from build123d import *

# Parameters (mm, degrees)
EXTRUDE_1_DEPTH = 2
FILLET_1_R      = 2


with BuildPart() as part:
    # 草图1 → 凸台-拉伸1 (new body)
    with BuildSketch(Plane.XY):
        Polygon((-8.301811847, -11.701358885), (-3.301811847, -11.701358885), (-3.301811847, -41.701358885), (13.698188153, -41.701358885), (13.698188153, -9.223166137), (34.95900929, -9.223166137), (34.95900929, 9.348641115), (13.698188153, 9.348641115), (7.098188153, 17.348641115), (-3.301811847, 17.348641115), (-3.301811847, 9.348641115), (0.698188153, 9.348641115), (0.698188153, 10.798641115), (3.898188153, 10.798641115), (3.898188153, 9.348641115), (7.098188153, 9.348641115), (7.098188153, 5.248641115), (3.898188153, 5.248641115), (3.898188153, 3.798641115), (0.698188153, 3.798641115), (0.698188153, 5.248641115), (-3.301811847, 5.248641115), (-3.301811847, -3.701358885), (-8.301811847, -3.701358885), align=None)
        with BuildLine():
            Line((0.698188153, -25.451358885), (8.698188153, -25.451358885))
            ThreePointArc((8.698188153, -25.451358885), (9.948188153, -26.701358885), (8.698188153, -27.951358885))
            Line((8.698188153, -27.951358885), (0.698188153, -27.951358885))
            ThreePointArc((0.698188153, -27.951358885), (-0.551811847, -26.701358885), (0.698188153, -25.451358885))
        make_face(mode=Mode.SUBTRACT)
        with BuildLine():
            Line((8.698188153, -37.451358885), (0.698188153, -37.451358885))
            ThreePointArc((0.698188153, -37.451358885), (-0.551811847, -36.201358885), (0.698188153, -34.951358885))
            Line((0.698188153, -34.951358885), (8.698188153, -34.951358885))
            ThreePointArc((8.698188153, -34.951358885), (9.948188153, -36.201358885), (8.698188153, -37.451358885))
        make_face(mode=Mode.SUBTRACT)
        with BuildLine():
            Line((32.20900929, 3.348641115), (32.20900929, -4.651358885))
            ThreePointArc((32.20900929, -4.651358885), (30.95900929, -5.901358885), (29.70900929, -4.651358885))
            Line((29.70900929, -4.651358885), (29.70900929, 3.348641115))
            ThreePointArc((29.70900929, 3.348641115), (30.95900929, 4.598641115), (32.20900929, 3.348641115))
        make_face(mode=Mode.SUBTRACT)
        with BuildLine():
            Line((22.70900929, 3.348641115), (22.70900929, -4.651358885))
            ThreePointArc((22.70900929, -4.651358885), (21.45900929, -5.901358885), (20.20900929, -4.651358885))
            Line((20.20900929, -4.651358885), (20.20900929, 3.348641115))
            ThreePointArc((20.20900929, 3.348641115), (21.45900929, 4.598641115), (22.70900929, 3.348641115))
        make_face(mode=Mode.SUBTRACT)
    extrude(amount=EXTRUDE_1_DEPTH)

    # 圆角1
    fillet_1_edges = [part.edges().sort_by_distance(p)[0] for p in [
        (-8.301811847, -3.701358885, 1),
        (-8.301811847, -11.701358885, 1),
    ]]
    fillet(fillet_1_edges, radius=FILLET_1_R)


solid = part.part
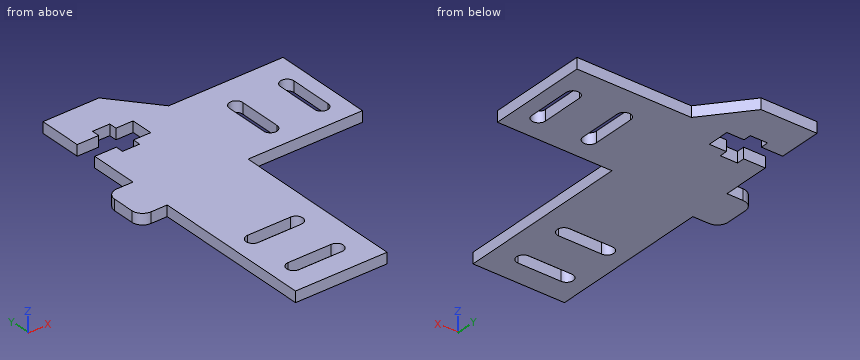
For this review, take the finished solid that the model builds, in its own axes (mm). Round coordinates to 2 decimals unless told otherwise and drop trailing zeros. Write each loop counter-clockwise with the first axis right and the second up, starting at its lowest first coordinate (ties: lowest second). Pieces come first, ordered by that corner, then holes. Notation, with made-up numbers: (16.25, 25) - (20.25, 25) arc R23 ccw to (20.25, 64) - close; hole circle Ø1 at (85, -30). An arc over 180 degrees is marked (long way). Use a Markdown table: item, result.
Q1. We need section D-D (y = -23.5). Give the boundary of the cut face in (x, z).
Derived:
| item | result |
|---|---|
| outline | (-3.3, 0) - (13.7, 0) - (13.7, 2) - (-3.3, 2) - close |
Q2. Clearance check with flat-ended pins moving along their axes: pin 1 (1.2 mm diameter, centred on y = 10, z = 1, fed in from -X); pin 2 (1.5 mm diameter, centred on x = 0.5, y = 8.5, fed in from +Z); pin 3 (1 mm diameter, centred on x = -5, z = 0.5, fed in from +Y). State where each tip first meets the part, or that it passes through.
Derived:
| item | result |
|---|---|
| pin 1 | stops at x = -3.3 |
| pin 2 | passes through |
| pin 3 | stops at y = -3.7 |
Q3. We need section B-B (z = 1.45). State how many separate pieces and enclosed holes the cut face has, plus the area to 3 significant figures.
Derived:
| item | result |
|---|---|
| separate pieces | 1 |
| enclosed holes | 4 |
| area | 1,260 mm2 |
Q4. Wall thickness on line 1 along X through (y, z) = (1.5, 1.1); line 2 along Y through (x, z) = (6, 1.6); line 3 along X through (y, z) = (-5.5, 1.7): over which ranges is each line inside the solid? List them lowest first.
Derived:
| item | result |
|---|---|
| line 1 | x = -3.3 to 20.21, 22.71 to 29.71, 32.21 to 34.96 |
| line 2 | y = -41.7 to -37.45, -34.95 to -27.95, -25.45 to 5.25, 9.35 to 17.35 |
| line 3 | x = -8.29 to 20.54, 22.38 to 30.04, 31.88 to 34.96 |
Q5. We need section C-C (x = 28). Give the boundary of the cut face in (y, z), plus the area to 3 significant figures.
Derived:
| item | result |
|---|---|
| outline | (-9.22, 0) - (9.35, 0) - (9.35, 2) - (-9.22, 2) - close |
| area | 37.1 mm2 |
Q6. We need section A-A (x = -1.5). Give the boundary of the cut face in (y, z), plus the area to 3 significant figures.
Derived:
| item | result |
|---|---|
| outline | (-41.7, 0) - (5.25, 0) - (5.25, 2) - (-41.7, 2) - close; (9.35, 0) - (17.35, 0) - (17.35, 2) - (9.35, 2) - close |
| area | 110 mm2 |
